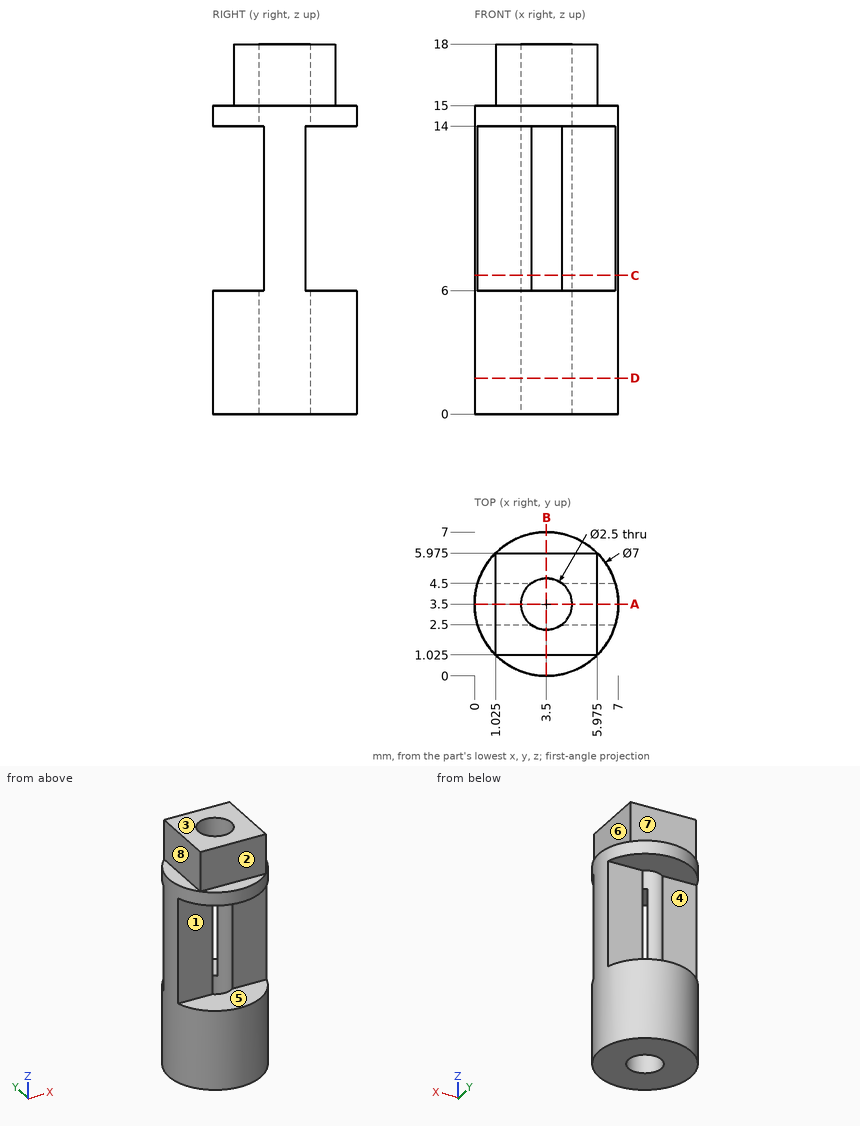
Drawing for the job (mm, zero at the part's lowest x, y, z). A direction names the side the tool comes from. Coordinates: 2 decimals unless noted, no trailing zeros. Write each loop counter-clockwise with the first axis right and the second up, starting at its lowest first coordinate (ties: lowest second). Pieces come first, ordered by that corner, then holes. Notation, with made-up numbers: (85, 28) -> (108, 28) arc R25 cw to (108, 47) -> close; hole circle Ø8 at (-36.75, 66.5). An arc over 180 degrees is marked (long way). One line per item, written item: value. Start each with the question number.
1) Which spindle directions (+Z, -Z, +X, -X, +Y, -Y) get a long thin tool onto all of the face, cutting with end or side? Do the marked faces 4, 5, 6, 7 and 8. Say none if no direction does.
2) Pull direction Z, two halves, no side cores. Call the marked faces 1, 2 and 3: +Z half, -Z half, draft (parallel to the pull), parting line (faces both ways), or undercut.
3) Probe probe 1 along Y at (x, z) = (3.5, 4.5); probe 2 along Z at (x, y) = (4, 2); probe 3 along Y at (x, z) = (5, 6.25). List the from-to ranges inside material, lowest first.
4) Slice it at D-D on z = 1.75. Write the cut outline in (x, y), then the cut area to 3 significant figures.
5) Flat gauge pins, fed straight in: pin 1 Ø2.5 at (x, z) = (4.5, 17) entering from -Y (3 decimals); pin 2 Ø2 at (y, z) = (1, 5) entering from +X; pin 3 Ø1.5 at (x, y) = (3.5, 3.5) entering from -Z; pin 4 Ø0.8 at (x, y) = (2.5, 0.5) entering from +Z. Where does each tip first touch, or does it go through?
6) Slice it at C-C on z = 6.75. Write the cut outline in (x, y).
7) Slice it at B-B on x = 3.5. Write the cut outline in (y, z) (3 decimals).
8) Slice it at A-A on y = 3.5. Write the cut outline in (x, z) (3 decimals).
Answers follow:
1. face 4: +X, -X, +Y
1. face 5: +X, -X, -Y
1. face 6: +Z, +X, +Y, -Y
1. face 7: +Z, +X, -X, +Y
1. face 8: +Z, -X, +Y, -Y
2. face 1: undercut
2. face 2: draft
2. face 3: +Z half
3. probe 1: 0 to 2.25, 4.75 to 7
3. probe 2: 0 to 6, 14 to 18
3. probe 3: 2.5 to 4.5
4. outline: circle Ø7 at (3.5, 3.5); hole circle Ø2.5 at (3.5, 3.5)
4. area: 33.6 mm2
5. pin 1: y = 1.025
5. pin 2: x = 6.66
5. pin 3: through
5. pin 4: z = 15
6. outline: (0.15, 2.5) -> (2.75, 2.5) arc R1.25 cw to (2.75, 4.5) -> (0.15, 4.5) arc R3.5 ccw to start; (4.25, 2.5) -> (6.85, 2.5) arc R3.5 ccw to (6.85, 4.5) -> (4.25, 4.5) arc R1.25 cw to start
7. outline: (0, 0) -> (2.25, 0) -> (2.25, 6) -> (0, 6) -> close; (0, 14) -> (2.25, 14) -> (2.25, 18) -> (1.025, 18) -> (1.025, 15) -> (0, 15) -> close; (4.75, 0) -> (7, 0) -> (7, 6) -> (4.75, 6) -> close; (4.75, 14) -> (7, 14) -> (7, 15) -> (5.975, 15) -> (5.975, 18) -> (4.75, 18) -> close
8. outline: (0, 0) -> (2.25, 0) -> (2.25, 18) -> (1.025, 18) -> (1.025, 15) -> (0, 15) -> close; (4.75, 0) -> (7, 0) -> (7, 15) -> (5.975, 15) -> (5.975, 18) -> (4.75, 18) -> close
